Part model, mm, in its own coordinate system. A direction names the side the tool comes from. Give positions to 0.01 mm unless a question says otherwise; leave off trailing zeros. Order: outer loops, then holes, each group sorted by start corner. A loop starts at its lowest first (then second) coordinate and runs counter-clockwise, first axis right, second up. Notation, with made-up numbers: (78, -14) -> (93, -14) arc R16 ccw to (93, 17) -> close; hole circle Ø6 at (35, 46.25). An arc over 180 degrees is marked (long way). Write item = value, one per line. Start each with the question number.
(1) Flat gauge pins, fed straight in: pin 1 (0.9 mm diameter, centred on x = 19, y = 2, fed in from -Z); pin 2 (7 mm diameter, centred on x = 0, z = 0, fed in from +Y); pin 3 (0.9 mm diameter, centred on y = 1, z = 19.5, fed in from -X); pin 4 (2 mm diameter, centred on x = 14, z = 18.5, fed in from +Y). Where does each tip first touch, or does it go through?
(2) Two-plate mould, pull along X, no slides. Class faces 1 (the flat face through (21.899, 1.521, 1.213)), 2 (the flat face through (18, 2, 12)), 3 (the flat face through (-6, 2, 0)): pulls with the +X half, pulls with the -X half, needs draft (parallel to the pull), parting line crosses it, or undercut.
(3) Saw through at C-C, the plane x = -13. List the corners of the cut face in (y, z).
(4) Saw through at B-B, the plane y = 1. State how many separate pieces and enclosed holes the cut face has, then the cut area to 3 significant figures.
(5) Probe line 1 along X through (y, z) = (0.5, 4.5); line 2 along Z through (x, y) = (-21.5, 1.8); line 3 along X through (y, z) = (0.2, 3.5). List the from-to ranges inside material, lowest first. Write a range as from..to.
(6) Saw through at A-A, the plane z = 1.5. List the corners of the cut face in (x, y).
(7) Which spindle directions (+Z, -Z, +X, -X, +Y, -Y) get a long thin tool onto all of the face, cutting with end or side? Do faces 4 (the flat face through (-14.69, 1.52, 16.36)), 5 (the flat face through (-19.57, 1.52, 9.9)), 6 (the flat face through (9.957, 1.521, -19.605)), 7 (the flat face through (20.904, 1.521, -6.822)). Say none if no direction does.
from build123d import *

# Parameters (mm, degrees)
SKETCH1_R           = 20
BOSS_EXTRUDE1_DEPTH = 3
BOSS_EXTRUDE2_DEPTH = 3
CIRPATTERN1_COUNT   = 24
SKETCH3_R           = 3
CUT_EXTRUDE1_DEPTH  = 3
SKETCH4_W           = 3
SKETCH4_H           = 10
CUT_EXTRUDE2_DEPTH  = 10


with BuildPart() as part:
    # Sketch1 → Boss-Extrude1 (new body)
    with BuildSketch(Plane(origin=(0, 0, 0), x_dir=(1, 0, 0), z_dir=(0, 1, 0))):
        with Locations(Location((0, 0, 0), (0, 0, 270))):
            Circle(SKETCH1_R)
    extrude(amount=BOSS_EXTRUDE1_DEPTH)

    # Sketch2 → Boss-Extrude2 (add)
    with BuildSketch(Plane(origin=(0, 3, 0), x_dir=(1, 0, 0), z_dir=(0, 1, 0))):
        Polygon((0, 24), (-2.392304845, 19.856406461), (2.392304845, 19.856406461), align=None)
    boss_extrude2 = extrude(amount=-BOSS_EXTRUDE2_DEPTH)

    # CirPattern1: Boss-Extrude2 ×24 about axis
    cirpattern1_axis = Axis((0, 0, 0), (0, 1, 0))
    for i in range(1, CIRPATTERN1_COUNT):
        add(boss_extrude2.rotate(cirpattern1_axis, i * 360 / CIRPATTERN1_COUNT))

    # Sketch3 → Cut-Extrude1 (cut)
    with BuildSketch(Plane(origin=(0, 3, 0), x_dir=(1, 0, 0), z_dir=(0, 1, 0))):
        with Locations(Location((0, 0, 0), (0, 0, 270))):
            Circle(SKETCH3_R)
    extrude(amount=-CUT_EXTRUDE1_DEPTH, mode=Mode.SUBTRACT)

    # Sketch4 → Cut-Extrude2 (cut)
    with BuildSketch(Plane(origin=(0, 3, 0), x_dir=(1, 0, 0), z_dir=(0, 1, 0))):
        with Locations((-7.5, 0)):
            Rectangle(SKETCH4_W, SKETCH4_H)
        with Locations((7.5, 0)):
            Rectangle(SKETCH4_W, SKETCH4_H)
    extrude(amount=-CUT_EXTRUDE2_DEPTH, mode=Mode.SUBTRACT)


solid = part.part
Results list:
q1.pin_1 = -12
q1.pin_2 = 3
q1.pin_3 = -12
q1.pin_4 = through
q2.face_1 = pulls with the +X half
q2.face_2 = needs draft
q2.face_3 = undercut
q3.outline = (0, -15.91) -> (3, -15.91) -> (3, 15.91) -> (0, 15.91) -> close
q4.separate_pieces = 1
q4.enclosed_holes = 3
q4.area = 1,400 mm^2
q5.line_1 = -21.47..-9, -6..6, 9..21.47
q5.line_2 = -6.66..-4.53, -1.44..1.44, 4.53..6.66
q5.line_3 = -20.47..-9, -6..6, 9..20.47
q6.outline = (-21.4, 0) -> (-9, 0) -> (-9, 3) -> (-21.4, 3) -> close; (-6, 0) -> (-2.6, 0) -> (-2.6, 3) -> (-6, 3) -> close; (2.6, 0) -> (6, 0) -> (6, 3) -> (2.6, 3) -> close; (9, 0) -> (21.4, 0) -> (21.4, 3) -> (9, 3) -> close
q7.face_4 = +Z, +Y, -Y
q7.face_5 = -X, +Y, -Y
q7.face_6 = -Z, +Y, -Y
q7.face_7 = +X, +Y, -Y
